Check sheet for the modelled part. Datum: model origin and axes. Units: mm. Face numbers are marked on the shaded views. A direction names the side the tool comes from. Coordinates: 2 decimals unless noted, no trailing zeros. Loops run counter-clockwise (first coordinate to the right, second up) from the corner with the lowest first, then second, coordinate; pieces in that order, holes last. Notation, with made-up numbers: (-23, 25.5) -> (36, 25.5) arc R15 ccw to (36, 35.5) -> close; hole circle Ø8 at (58, 57). An arc over 180 degrees is marked (long way). Use one line per item in the form item = value.
from build123d import *

# Parameters (mm, degrees)
BOSS_EXTRUDE1_DEPTH = 12.7
BOSS_EXTRUDE2_DEPTH = 38.1
FILLET1_R           = 25.4
FILLET2_R           = 20.32
FILLET3_R           = 6.35
FILLET4_R           = 1.2699999999999994
CUT_EXTRUDE1_DEPTH  = 38.1
SKETCH5_R           = 6.826249999999999
SKETCH5_R_2         = 6.826250000000001
CUT_EXTRUDE4_DEPTH  = 20.32


with BuildPart() as part:
    # Sketch1 → Boss-Extrude1 (new body)
    with BuildSketch(Plane(origin=(0, 0, 0), x_dir=(1, 0, 0), z_dir=(0, 1, 0))):
        Polygon((39.86388888888888, 22.225000000000012), (-39.86388888888888, 22.225), (-28.574999999999996, -28.57499999999998), (28.575000000000006, -28.574999999999978), align=None)
        Polygon((41.27499999999999, 28.575000000000014), (-41.275000000000006, 28.575000000000003), (-39.863888888888894, 22.225), (39.86388888888888, 22.225000000000012), align=None)
    extrude(amount=BOSS_EXTRUDE1_DEPTH)

    # Sketch1<5> → Boss-Extrude2 (add)
    with BuildSketch(Plane(origin=(0, 0, 0), x_dir=(1, 0, 0), z_dir=(0, 1, 0))):
        Polygon((41.27499999999999, 28.575000000000014), (-41.275000000000006, 28.575000000000003), (-39.863888888888894, 22.225), (39.86388888888888, 22.225000000000012), align=None)
    extrude(amount=BOSS_EXTRUDE2_DEPTH)

    # Fillet1
    fillet1_edges = [part.edges().sort_by_distance(p)[0] for p in [
        (0, 12.7, -22.22500000000001),
    ]]
    fillet(fillet1_edges, radius=FILLET1_R - 0.0001)  # a hair under: the kernel refuses the full size

    # Fillet2
    fillet2_edges = [part.edges().sort_by_distance(p)[0] for p in [
        (28.575000000000006, 6.35, 28.574999999999978),
        (-28.574999999999996, 6.35, 28.57499999999998),
    ]]
    fillet(fillet2_edges, radius=FILLET2_R)

    # Fillet3
    fillet3_edges = [part.edges().sort_by_distance(p)[0] for p in [
        (-7.11e-15, 0, -28.57500000000001),
    ]]
    fillet(fillet3_edges, radius=FILLET3_R)

    # Fillet4
    fillet4_edges = [part.edges().sort_by_distance(p)[0] for p in [
        (0, 38.1, -22.22500000000001),
        (-7.11e-15, 38.1, -28.57500000000001),
    ]]
    fillet(fillet4_edges, radius=FILLET4_R)

    # Sketch4 → Cut-Extrude1 (cut)
    with BuildSketch(Plane(origin=(-3.6e-15, 0, -28.57500000000001), x_dir=(-1, 0, 1.3e-16), z_dir=(-1.3e-16, 0, -1))):
        with BuildLine():
            ThreePointArc((-22.35199999999955, 28.703096211960737), (-18.92299999999955, 25.27409621196074), (-15.493999999999552, 28.703096211960737))
            Line((-15.493999999999552, 28.70309621196053), (-22.35199999999955, 28.70309621196053))
        make_face()
        with BuildLine():
            Line((-22.35199999999955, 28.70309621196053), (-15.493999999999552, 28.70309621196053))
            ThreePointArc((-15.493999999999552, 28.703096211960737), (-18.92299999999955, 32.132096211960736), (-22.35199999999955, 28.703096211960737))
        make_face()
        with BuildLine():
            ThreePointArc((15.748000000000676, 28.70309621196054), (19.177000000000678, 25.274096211960536), (22.60600000000068, 28.70309621196054))
            Line((22.60600000000068, 28.703096211960535), (15.748000000000676, 28.703096211960535))
        make_face()
        with BuildLine():
            Line((15.748000000000676, 28.703096211960535), (22.60600000000068, 28.703096211960535))
            ThreePointArc((22.60600000000068, 28.70309621196054), (19.177000000000678, 32.132096211960544), (15.748000000000676, 28.70309621196054))
        make_face()
    extrude(amount=-CUT_EXTRUDE1_DEPTH, mode=Mode.SUBTRACT)

    # Sketch5 → Cut-Extrude4 (cut)
    with BuildSketch(Plane(origin=(-2.8e-15, 0, -22.22500000000001), x_dir=(-1, 0, 1.3e-16), z_dir=(-1.3e-16, 0, -1))):
        with Locations((-18.92299999999955, 28.703096211960737)):
            Circle(SKETCH5_R)
        with Locations((19.177000000000678, 28.70309621196054)):
            Circle(SKETCH5_R_2)
    extrude(amount=-CUT_EXTRUDE4_DEPTH, mode=Mode.SUBTRACT)


solid = part.part
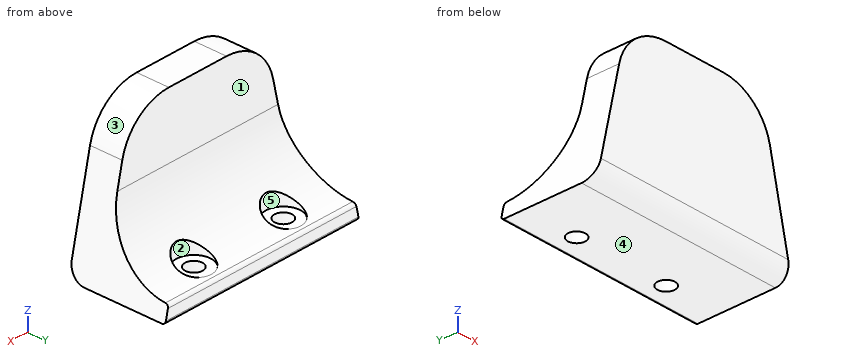
(1) Mould release check, pull along Y, two halves, no side actions. Record for the marked faces 1, 2 and 3: +Y half, -Y half, draft (parallel to the pull), parting line (faces both ways), or undercut.
Established:
face_1 = +Y half
face_2 = undercut
face_3 = draft
(2) Tool access check on the marked faces 4 and 5. Record the directions out of +Z, -Z, +X, -X, +Y, -Y that give a thin tool (end or side, any length) a straight path to the whole face; none if there is none.
Established:
face_4 = -Z, +X, -X, +Y, -Y
face_5 = +Z
(3) Section check B-B, the plane y = 30. Record the boundary of the cut face in (x, z) (3 decimals), plus the area to 3 significant figures.
Established:
outline = (-41.275, -28.575) -> (-22.351, -28.575) -> (-22.351, -22.225) -> (-25.879, -22.225) -> (-25.879, -20.899) -> (-39.569, -20.899) -> close; (-16.003, -28.575) -> (15.749, -28.575) -> (15.749, -22.225) -> (12.221, -22.225) -> (12.221, -20.899) -> (-12.475, -20.899) -> (-12.475, -22.225) -> (-16.003, -22.225) -> close; (22.097, -28.575) -> (41.275, -28.575) -> (39.569, -20.899) -> (25.625, -20.899) -> (25.625, -22.225) -> (22.097, -22.225) -> close
area = 504 mm²
(4) Section check C-C, the plane z = -17.5. Record the boundary of the cut face in (x, y), plus the area to 3 significant figures.
Established:
outline = (-38.81, 0) -> (38.81, 0) -> (38.81, 23.35) -> (23.15, 23.35) arc R6.83 cw to (14.69, 23.35) -> (-14.95, 23.35) arc R6.83 cw to (-23.41, 23.35) -> (-38.81, 23.35) -> close
area = 1,800 mm²
(5) Scan lines: line 1 along Y through (x, z) = (31.5, 10.5); line 2 along Z through (x, y) = (-28.5, 18) (3 decimals); line 3 along Y through (x, z) = (21, -11). Record each from-to range of solid material in increasing order.
Established:
line_1 = 0 to 12.7
line_2 = -28.575 to -12.354
line_3 = 0 to 17.02
(6) Go/stop test with flat-tipped pins: P1, Ø10, axis at x = -10.5, z = 3, coming from the +Y side; P2, Ø12.5, axis at x = -11, z = 13, coming from the +Y side; P3, Ø6, axis at y = 22.5, z = -17, coming from the -X side; P4, Ø4, axis at x = -19.18, y = 28.7, coming from the -Z side. Record where each tip stops, or that it passes through.
Established:
P1 = 13.23
P2 = 12.7
P3 = -39.37
P4 = through
(7) Section check D-D, the plane y = 4. Record the boundary of the cut face in (x, z) (3 decimals), plus the area to 3 significant figures.
Established:
outline = (-41.175, -28.124) -> (41.175, -28.124) -> (32.111, 12.663) arc R20.32 ccw to (12.275, 28.575) -> (-12.275, 28.575) arc R20.32 ccw to (-32.111, 12.663) -> close
area = 3,850 mm²
(8) Section check A-A, the plane y = 10. Record the boundary of the cut face in (x, z) (3 decimals), plus the area to 3 significant figures.
Established:
outline = (-41.275, -28.575) -> (41.275, -28.575) -> (32.111, 12.663) arc R20.32 ccw to (12.275, 28.575) -> (-12.275, 28.575) arc R20.32 ccw to (-32.111, 12.663) -> close
area = 3,890 mm²
